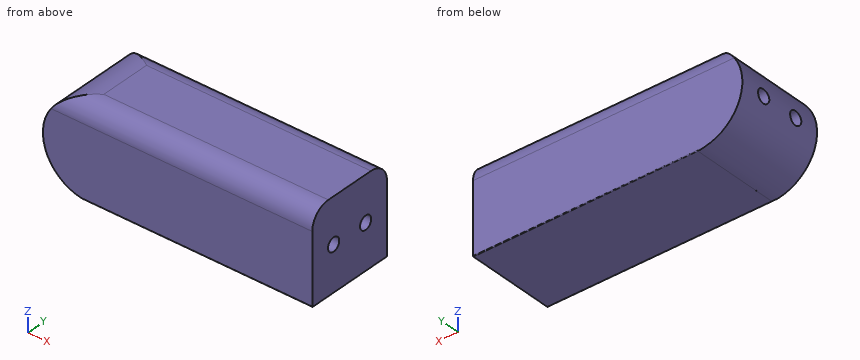
```python
from build123d import *

# Parameters (mm, degrees)
SKETCH1_R           = 69.995
SKETCH1_W           = 350
SKETCH1_H           = 140
BOSS_EXTRUDE1_DEPTH = 140
SKETCH2_R           = 10.5
CUT_EXTRUDE3_DEPTH  = 41
FILLET2_R           = 30
FILLET3_R           = 1
CUT_EXTRUDE4_START  = -41
SKETCH3_R           = 10.5
CUT_EXTRUDE4_DEPTH  = 41


with BuildPart() as part:
    # Sketch1 → Boss-Extrude1 (new body)
    with BuildSketch(Plane(origin=(0, 0, 0), x_dir=(1, 0, 0), z_dir=(0, 1, 0))):
        with Locations((0, -70)):
            Circle(SKETCH1_R)
        with Locations((175, -70)):
            Rectangle(SKETCH1_W, SKETCH1_H)
    extrude(amount=BOSS_EXTRUDE1_DEPTH)

    # Sketch2 → Cut-Extrude3 (cut)
    with BuildSketch(Plane(origin=(-70, 0, 0), x_dir=(0, 0, -1), z_dir=(1, 0, 0))):
        with Locations(Location((-70, 100, 0), (0, 0, 180))):
            Circle(SKETCH2_R)
        with Locations(Location((-70, 40, 0), (0, 0, 180))):
            Circle(SKETCH2_R)
    extrude(amount=CUT_EXTRUDE3_DEPTH, mode=Mode.SUBTRACT)

    # Fillet2
    fillet2_edges = [part.edges().sort_by_distance(p)[0] for p in [
        (175, 140, 140),
        (175, 0, 140),
    ]]
    fillet(fillet2_edges, radius=FILLET2_R)

    # Fillet3
    fillet3_edges = [part.edges().sort_by_distance(p)[0] for p in [
        (175, 140, 0),
        (175, 0, 0),
    ]]
    fillet(fillet3_edges, radius=FILLET3_R)

    # Sketch3 → Cut-Extrude4 (cut)
    with BuildSketch(Plane(origin=(350, 0, 0), x_dir=(0, 0, -1), z_dir=(1, 0, 0)).offset(CUT_EXTRUDE4_START)):
        with Locations(Location((-70, 100, 0), (0, 0, 180))):
            Circle(SKETCH3_R)
        with Locations(Location((-70, 40, 0), (0, 0, 180))):
            Circle(SKETCH3_R)
    extrude(amount=CUT_EXTRUDE4_DEPTH, mode=Mode.SUBTRACT)


solid = part.part
```
For this review, take the finished solid that the model builds, in its own axes (mm). Round coordinates to 2 decimals unless told otherwise and drop trailing zeros. Write each loop counter-clockwise with the first axis right and the second up, starting at its lowest first coordinate (ties: lowest second). Pieces come first, ordered by that corner, then holes. Notation, with made-up numbers: M 64,10 L 92,10 A30 ccw 92,45 Z; hole C -25.5,8.5 d6. An arc over 180 degrees is marked long. One line per item, written item: value. Start each with the question number.
(1) We need section B-B (z = 70). Give the boundary of the cut face in (x, y) (3 decimals), and give its area (3 significant figures).
(2) We need section C-C (y = 61.5). Give the boundary of the cut face in (x, z) (3 decimals), and give its area (3 significant figures).
(3) Insertion check: pin 1 (6.5 mm diameter, centred on y = 103, z = 74.5, fed in from +X); pin 2 (12.5 mm diameter, centred on y = 100, z = 70, fed in from -X); pin 3 (4 mm diameter, centred on x = 146, y = 22.5, fed in from +Z). Each pin has a flat end and moves straight along its axis. Give the tip position at first contact, or say it passes through.
(4) Wall thickness on line 1 (Y direction, x = 336.5, z = 70); line 2 (Z direction, x = 328, y = 100); line 3 (Z direction, x = 331, y = 97): over which ranges is each line inside the solid? List them lowest first.
(5) We need section A-A (x = 226.5). Give the boundary of the cut face in (y, z).
Result:
1. outline: M -69.995,0 L 350,0 L 350,29.5 L 309,29.5 L 309,50.5 L 350,50.5 L 350,89.5 L 309,89.5 L 309,110.5 L 350,110.5 L 350,140 L -69.995,140 L -69.995,110.5 L -29,110.5 L -29,89.5 L -69.995,89.5 L -69.995,50.5 L -29,50.5 L -29,29.5 L -69.995,29.5 Z
1. area: 55,400 mm²
2. outline: M 0,0 L 350,0 L 350,140 L 0,140 L 0,139.995 A69.995 ccw 0,0.005 Z
2. area: 56,700 mm²
3. pin 1: x = 309
3. pin 2: x = -29
3. pin 3: z = 139.49
4. line 1: 0 to 29.5, 50.5 to 89.5, 110.5 to 140
4. line 2: 0 to 59.5, 80.5 to 140
4. line 3: 0 to 59.94, 80.06 to 140
5. outline: M 0,1 A1 ccw 1,0 L 139,0 A1 ccw 140,1 L 140,110 A30 ccw 110,140 L 30,140 A30 ccw 0,110 Z
